Could you check a few things on this model? Use its own coordinates, in mm. Round coordinates to 2 decimals unless told otherwise and drop trailing zeros. Loops run counter-clockwise (first coordinate to the right, second up) from the corner with the lowest first, then second, coordinate; pieces in that order, holes last. Notation, with made-up numbers: (-29.5, -7.75) -> (-6.5, -7.75) arc R31 ccw to (-6.5, 29.25) -> close; hole circle Ø5 at (-19.75, 86.25). An arc over 180 degrees is marked (long way). Use CSV: the item, a comma, the result in double quotes. Start each with the question number.
Autodesk Inventor part; units mm, degrees
ref_plane "YZ Plane" through (0, 0, 0) normal (1, 0, 0) x (0, 1, 0)
ref_plane "XZ Plane" through (0, 0, 0) normal (0, 1, 0) x (-1, 0, 0)
ref_plane "XY Plane" through (0, 0, 0) normal (0, 0, 1) x (1, 0, 0)
sketch "Sketch1" plane through (0, 0, 0) normal (0, 0, 1) x (1, 0, 0)
  line L0 (0, 0) -> (14, 0) construction
  line L1 (14, 0) -> (14, 38.55) construction
  line L2 (14, 38.55) -> (0, 38.55)
  line L3 (0, 38.55) -> (0, 0) construction
  line L4 (0, 38.55) -> (0, 87.5)
  line L5 (0, 87.5) -> (14, 87.5)
  line L6 (14, 87.5) -> (14, 38.55)
  dimension "d1" = 14
  dimension "d2" = 77.1
  dimension "d3" = 175
revolve "Revolution1" add sketch "Sketch1" angle 360 about axis through (0, 0, 0) along (1, 0, 0)
sketch "Sketch2" plane through (14, 0, 0) normal (1, 0, 0) x (0, 0, -1)
  circle A0 centre (0, 0) radius 87.5
  circle A1 centre (-49.4975, 49.4975) radius 7.5
  circle A2 centre (0, 0) radius 70 construction
  line L0 (-49.4975, 49.4975) -> (0, 0) construction
  circle A3 centre (0, 0) radius 38.55
  line L1 (0, 0) -> (-70, 0) construction
  dimension "d5" = 140
  dimension "d6" = 15
  dimension "d12" = 45
extrude "Extrusion1" cut sketch "Sketch2" against normal through all contours A1
pattern_circular "Circular Pattern1" count 4 over 360 about axis through (7, 0, 0) along (1, 0, 0) of "Extrusion1"
equation "\"d5\" = C1"
equation "\"d6\" = h1"
equation "\"d1\" = t"
equation "\"d2\" = d0"
equation "\"d3\" = D"
equation "\"d0\" = 77.1"
equation "\"D\" = 175"
equation "\"t\" = 14"
equation "\"C1\" = 140"
equation "\"h1\" = 15"
properties part number "JIS B 2220 Slip-On Welding Thin Plate Type Flange SOP - 10K 65" material "Steel"
1. Suppose I cut it at C-C (y = -46). List the corners of the cut face in (x, z) for me.
2. Suppose I cut it at B-B (y = 30). List the corners of the cut face in (x, z) for me, then the cut area to 3 significant figures.
3. If I drill on L1, parallel to Z at x = 6.75, y = 47.5; L2, parallel to Y at x = 12, z = -56; L3, parallel to Y at x = 10.5, z = -1, over which ranges is the centre line in solid material (lowest first)?
4. We'd pull the mould along Z, two halves only. Please class faces 1 (the face through (0, 18, -38)), 2 (the face through (7.1, -56.99, 49.83)), 3 (the face through (7.1, -64.49, 59.14)): pulls with the +Z half, pulls with the -Z half, needs draft (parallel to the pull), parting line crosses it, or undercut.
5. Suppose I cut it at A-A (z = 0). List the corners of the cut face in (x, y) for me, then the cut area to 3 significant figures.
6. Suppose I cut it at D-D (z = -53.5). List the corners of the cut face in (x, y) for me, then the cut area to 3 significant figures.
7. Will these pins go through, and if not, where does the flat tip stop? pin 1 (3 mm diameter, centred on x = 6, z = -37.5, fed in from +Y); pin 2 (3 mm diameter, centred on x = 6.5, z = -29, fed in from -Y); pin 3 (8 mm diameter, centred on x = 11, y = -25, fed in from +Z).
Geometry check:
1,outline,"(0, -74.43) -> (14, -74.43) -> (14, -56.13) -> (0, -56.13) -> close; (0, -42.86) -> (14, -42.86) -> (14, 42.86) -> (0, 42.86) -> close; (0, 56.13) -> (14, 56.13) -> (14, 74.43) -> (0, 74.43) -> close"
2,outline,"(0, -82.2) -> (14, -82.2) -> (14, -24.21) -> (0, -24.21) -> close; (0, 24.21) -> (14, 24.21) -> (14, 82.2) -> (0, 82.2) -> close"
2,area,"1,620 mm²"
3,L1,"z = -73.48 to -56.73, -42.27 to 42.27, 56.73 to 73.48"
3,L2,"y = -67.23 to -53.23, -45.76 to 45.76, 53.23 to 67.23"
3,L3,"y = -87.49 to -38.54, 38.54 to 87.49"
4,face 1,"needs draft"
4,face 2,"undercut"
4,face 3,"parting line crosses it"
5,outline,"(0, -87.5) -> (14, -87.5) -> (14, -38.55) -> (0, -38.55) -> close; (0, 38.55) -> (14, 38.55) -> (14, 87.5) -> (0, 87.5) -> close"
5,area,"1,370 mm²"
6,outline,"(0, -69.24) -> (14, -69.24) -> (14, -55.84) -> (0, -55.84) -> close; (0, -43.15) -> (14, -43.15) -> (14, 43.15) -> (0, 43.15) -> close; (0, 55.84) -> (14, 55.84) -> (14, 69.24) -> (0, 69.24) -> close"
6,area,"1,580 mm²"
7,pin 1,"stops at y = 79.75"
7,pin 2,"stops at y = -83.07"
7,pin 3,"stops at z = 84.94"
